from build123d import *

# Parameters (mm, degrees)
F0_R     = 2.3749
F1_DEPTH = 3.175
F3_DEPTH = 25.4


with BuildPart() as f1:
    # F0 (on Top) → F1 (new body)
    with BuildSketch(Plane.XY):
        with BuildLine():
            Line((-38.1, -9.525), (38.1, -9.525))
            Line((38.1, -9.525), (38.1, -1.905))
            ThreePointArc((38.1, -1.905), (36.612102, 1.687102), (33.02, 3.175))
            Line((33.02, 3.175), (9.243306, 3.175))
            ThreePointArc((9.243306, 3.175), (6.333003, 4.091283), (4.472567, 6.509591))
            ThreePointArc((4.472567, 6.509591), (0, 9.635769), (-4.472567, 6.509591))
            ThreePointArc((-4.472567, 6.509591), (-6.333003, 4.091283), (-9.243306, 3.175))
            Line((-9.243306, 3.175), (-33.02, 3.175))
            ThreePointArc((-33.02, 3.175), (-36.612102, 1.687102), (-38.1, -1.905))
            Line((-38.1, -1.905), (-38.1, -9.525))
        make_face()
        with Locations((0, 4.873269)):
            Circle(F0_R, mode=Mode.SUBTRACT)
    extrude(amount=F1_DEPTH)

    # F2 (on face) → F3 (cut)
    with BuildSketch(Plane.XY.offset(3.175)):
        Polygon((-38.1, -7.62), (-38.1, -14.148636), (38.1, -14.148636), (38.1, -7.62), (37.1475, -9.525), (36.195, -7.62), (35.2425, -9.525), (34.29, -7.62), (33.3375, -9.525), (32.385, -7.62), (31.4325, -9.525), (30.48, -7.62), (29.5275, -9.525), (28.575, -7.62), (27.6225, -9.525), (26.67, -7.62), (25.7175, -9.525), (24.765, -7.62), (23.8125, -9.525), (22.86, -7.62), (21.9075, -9.525), (20.955, -7.62), (20.0025, -9.525), (19.05, -7.62), (18.0975, -9.525), (17.145, -7.62), (16.1925, -9.525), (15.24, -7.62), (14.2875, -9.525), (13.335, -7.62), (12.3825, -9.525), (11.43, -7.62), (10.4775, -9.525), (9.525, -7.62), (8.5725, -9.525), (7.62, -7.62), (6.6675, -9.525), (5.715, -7.62), (4.7625, -9.525), (3.81, -7.62), (2.8575, -9.525), (1.905, -7.62), (0.9525, -9.525), (0, -7.62), (-0.9525, -9.525), (-1.905, -7.62), (-2.8575, -9.525), (-3.81, -7.62), (-4.7625, -9.525), (-5.715, -7.62), (-6.6675, -9.525), (-7.62, -7.62), (-8.5725, -9.525), (-9.525, -7.62), (-10.4775, -9.525), (-11.43, -7.62), (-12.3825, -9.525), (-13.335, -7.62), (-14.2875, -9.525), (-15.24, -7.62), (-16.1925, -9.525), (-17.145, -7.62), (-18.0975, -9.525), (-19.05, -7.62), (-20.0025, -9.525), (-20.955, -7.62), (-21.9075, -9.525), (-22.86, -7.62), (-23.8125, -9.525), (-24.765, -7.62), (-25.7175, -9.525), (-26.67, -7.62), (-27.6225, -9.525), (-28.575, -7.62), (-29.5275, -9.525), (-30.48, -7.62), (-31.4325, -9.525), (-32.385, -7.62), (-33.3375, -9.525), (-34.29, -7.62), (-35.2425, -9.525), (-36.195, -7.62), (-37.1475, -9.525), align=None)
    extrude(amount=-F3_DEPTH, mode=Mode.SUBTRACT)


solid = f1.part
Part model, mm, in its own coordinate system. Coordinates: 2 decimals unless noted, no trailing zeros. Use a Markdown table: item, result. Add a question column.
Item 1: Probe probe 1 along X at (y, z) = (4.25, 2.4); probe 2 along X at (y, z) = (8.5, 1.5); probe 3 along X at (y, z) = (-1.5, 1.2). List the from-to ranges inside material, lowest first.
Item 2: Flat gauge pins, fed straight in: P1, Ø3, axis at x = -10.5, y = 6, coming from the -Z side; P2, Ø1.6, axis at x = -21.5, z = 1.5, coming from the +Y side (3 decimals); P3, Ø1, axis at x = -4, z = 0.5, coming from the -Y side; P4, Ø1, axis at x = 30, y = -5, coming from the -Z side. Where does each tip first touch, or does it go through?
Item 3: Pull direction X, two halves, no side cores. Call faces 1 (the flat face through (-25.235, -8.559, 1.61)), 2 (the cylindrical face through (6.369, 4.067, 1.565)): +X half, -X half, draft (parallel to the pull), parting line (faces both ways), or undercut.
Geometry says:
| question | item | result |
|---|---|---|
| 1 | probe 1 | -6.12 to -2.29, 2.29 to 6.12 |
| 1 | probe 2 | -3.09 to 3.09 |
| 1 | probe 3 | -38.08 to 38.08 |
| 2 | P1 | through |
| 2 | P2 | y = 3.175 |
| 2 | P3 | y = -9 |
| 2 | P4 | z = 0 |
| 3 | face 1 | undercut |
| 3 | face 2 | +X half |
